The listing builds one solid part. Answer for the finished solid, in the listing's coordinates (mm). Face numbers are marked on the shaded views. A direction names the side the tool comes from. Coordinates: 2 decimals unless noted, no trailing zeros. Loops run counter-clockwise (first coordinate to the right, second up) from the corner with the lowest first, then second, coordinate; pieces in that order, holes last. Notation, with made-up numbers: (70, 34.5) -> (129, 34.5) arc R7 ccw to (129, 39.5) -> close; hole circle Ø6 at (-16, -29). An arc over 180 degrees is marked (long way). Answer in a Markdown table with one row per item.
```python
from build123d import *

# Parameters (mm, degrees)
BOSS_EXTRUDE1_DEPTH = 2.5
SKETCH2_R           = 1
CUT_EXTRUDE1_DEPTH  = 4.5
SKETCH3_R           = 1
CUT_EXTRUDE2_DEPTH  = 9.5
SKETCH5_R           = 1
BOSS_EXTRUDE2_DEPTH = 9.5
SKETCH7_W           = 2.5
SKETCH7_H           = 2.48697386
BOSS_EXTRUDE5_DEPTH = 17
SKETCH8_R           = 1
CUT_EXTRUDE3_DEPTH  = 9.5
SKETCH9_W           = 2.5
SKETCH9_H           = 2.510853282
CUT_EXTRUDE4_DEPTH  = 10.5
SKETCH10_R          = 1
CUT_EXTRUDE5_DEPTH  = 4.5
SKETCH11_R          = 1
BOSS_EXTRUDE6_DEPTH = 4.5
SKETCH12_R          = 1
CUT_EXTRUDE6_DEPTH  = 4
SKETCH13_W          = 2.5
SKETCH13_H          = 2.5
CUT_EXTRUDE7_DEPTH  = 6.5
SKETCH14_W          = 2.5
SKETCH14_H          = 2.5
BOSS_EXTRUDE7_DEPTH = 6.5
SKETCH15_R          = 1
CUT_EXTRUDE8_DEPTH  = 5


with BuildPart() as part:
    # Sketch1 → Boss-Extrude1 (new body)
    with BuildSketch(Plane.XY):
        Polygon((-70.406172668, -77.710060133), (-55.350496572, -77.710060133), (-55.155758053, -77.477979804), (-53.240646945, -79.084948828), (-54.184487309, -80.209773972), (-70.368347793, -80.209773972), align=None)
    extrude(amount=BOSS_EXTRUDE1_DEPTH)

    # Sketch2 → Cut-Extrude1 (cut)
    with BuildSketch(Plane(origin=(-60.939488189, -72.62485398, 0), x_dir=(0, 0, -1), z_dir=(0.6427876096865354, 0.7660444431189815, 0))):
        with Locations(Location((-1.25, -8.800123479, 0), (0, 0, 90))):
            Circle(SKETCH2_R)
    extrude(amount=-CUT_EXTRUDE1_DEPTH, mode=Mode.SUBTRACT)

    # Sketch3 → Cut-Extrude2 (cut)
    with BuildSketch(Plane(origin=(-71.565670343, -1.082908957, 0), x_dir=(0, 0, 1), z_dir=(-0.9998855357578962, -0.015129949839474955, 0))):
        with Locations(Location((1.25, -77.885923249, 0), (0, 0, 270))):
            Circle(SKETCH3_R)
    extrude(amount=-CUT_EXTRUDE2_DEPTH, mode=Mode.SUBTRACT)

    # Sketch5 → Boss-Extrude2 (add)
    with BuildSketch(Plane(origin=(-71.565670343, -1.082908957, 0), x_dir=(0, 0, 1), z_dir=(-0.9998855357578961, -0.015129949839476386, 0))):
        with Locations((1.25, -77.885923249)):
            Circle(SKETCH5_R)
    extrude(amount=-BOSS_EXTRUDE2_DEPTH)

    # Sketch7 → Boss-Extrude5 (add)
    with BuildSketch(Plane(origin=(-71.565670343, -1.082908957, 0), x_dir=(0, 0, 1), z_dir=(-0.9998855357578961, -0.015129949839476386, 0))):
        with Locations((1.25, -77.879410179)):
            Rectangle(SKETCH7_W, SKETCH7_H)
    extrude(amount=BOSS_EXTRUDE5_DEPTH)

    # Sketch8 → Cut-Extrude3 (cut)
    with BuildSketch(Plane(origin=(-88.56372445, -1.340118104, 0), x_dir=(0, 0, 1), z_dir=(-0.9998855357578962, -0.015129949839480206, 0))):
        with Locations(Location((1.25, -77.885923249, 0), (0, 0, 270))):
            Circle(SKETCH8_R)
    extrude(amount=-CUT_EXTRUDE3_DEPTH, mode=Mode.SUBTRACT)

    # Sketch9 → Cut-Extrude4 (cut)
    with BuildSketch(Plane(origin=(-88.56372445, -1.340118104, 0), x_dir=(0, 0, 1), z_dir=(-0.9998855357578962, -0.015129949839480206, 0))):
        with Locations((1.25, -77.89134989)):
            Rectangle(SKETCH9_W, SKETCH9_H)
    extrude(amount=-CUT_EXTRUDE4_DEPTH, mode=Mode.SUBTRACT)

    # Sketch10 → Cut-Extrude5 (cut)
    with BuildSketch(Plane(origin=(-78.064926325, -1.181253631, 0), x_dir=(0, 0, 1), z_dir=(-0.9998855357578961, -0.015129949839478678, 0))):
        with Locations(Location((1.25, -77.885923249, 0), (0, 0, 270))):
            Circle(SKETCH10_R)
    extrude(amount=-CUT_EXTRUDE5_DEPTH, mode=Mode.SUBTRACT)

    # Sketch11 → Boss-Extrude6 (add)
    with BuildSketch(Plane(origin=(-78.064926325, -1.181253631, 0), x_dir=(0, 0, 1), z_dir=(-0.9998855357578961, -0.015129949839478678, 0))):
        with Locations((1.25, -77.885923249)):
            Circle(SKETCH11_R)
    extrude(amount=-BOSS_EXTRUDE6_DEPTH)

    # Sketch12 → Cut-Extrude6 (cut)
    with BuildSketch(Plane(origin=(-78.064926325, -1.181253631, 0), x_dir=(0, 0, 1), z_dir=(-0.9998855357578961, -0.015129949839478678, 0))):
        with Locations(Location((1.25, -77.885923249, 0), (0, 0, 270))):
            Circle(SKETCH12_R)
    extrude(amount=-CUT_EXTRUDE6_DEPTH, mode=Mode.SUBTRACT)

    # Sketch13 → Cut-Extrude7 (cut)
    with BuildSketch(Plane(origin=(-78.064926325, -1.181253631, 0), x_dir=(0, 0, 1), z_dir=(-0.9998855357578961, -0.015129949839478678, 0))):
        with Locations((1.25, -77.885923249)):
            Rectangle(SKETCH13_W, SKETCH13_H)
    extrude(amount=-CUT_EXTRUDE7_DEPTH, mode=Mode.SUBTRACT)

    # Sketch14 → Boss-Extrude7 (add)
    with BuildSketch(Plane(origin=(-71.565670343, -1.082908957, 0), x_dir=(0, 0, 1), z_dir=(-0.9998855357578961, -0.015129949839476386, 0))):
        with Locations((1.25, -77.885923249)):
            Rectangle(SKETCH14_W, SKETCH14_H)
    extrude(amount=BOSS_EXTRUDE7_DEPTH)

    # Sketch15 → Cut-Extrude8 (cut)
    with BuildSketch(Plane(origin=(-78.064926325, -1.181253631, 0), x_dir=(0, 0, 1), z_dir=(-0.9998855357578961, -0.01512994983947622, 0))):
        with Locations(Location((1.25, -77.885923249, 0), (0, 0, 270))):
            Circle(SKETCH15_R)
    extrude(amount=-CUT_EXTRUDE8_DEPTH, mode=Mode.SUBTRACT)


solid = part.part
```
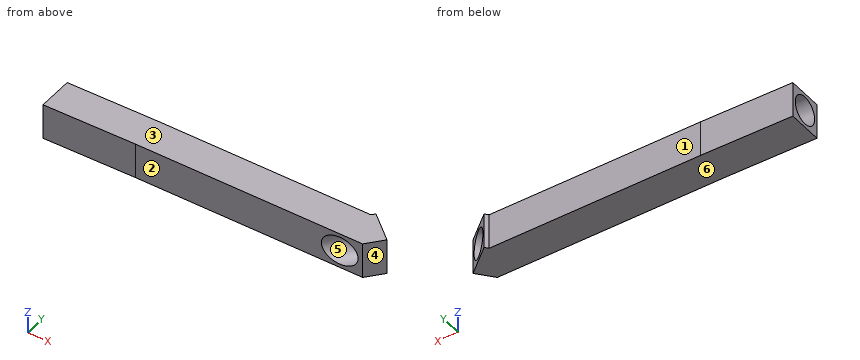
Item 1: A cutting plane is placed at C-C, the plane x = -71.25. Determine the outline of the cut face in (y, z), plus the area to 3 significant figures.
Findings below:
| item | result |
|---|---|
| outline | (-80.22, 0) -> (-77.72, 0) -> (-77.72, 2.5) -> (-80.22, 2.5) -> close |
| area | 6.25 mm2 |
Item 2: Find the intervals of material crossed by probe 1 along Y at (x, z) = (-61.5, 0.4); probe 2 along X at (y, z) = (-79.8, 0.4); probe 3 along X at (y, z) = (-79, 1.3), in increasing order.
Findings below:
| item | result |
|---|---|
| probe 1 | y = -80.21 to -77.71 |
| probe 2 | x = -76.88 to -56.16, -54.78 to -53.84 |
| probe 3 | x = -71.89 to -56.1, -53.5 to -53.34 |
Item 3: A cutting plane is placed at B-B, the plane x = -60.75. Determine the outline of the cut face in (y, z), plus the area to 3 significant figures.
Findings below:
| item | result |
|---|---|
| outline | (-80.21, 0) -> (-77.71, 0) -> (-77.71, 2.5) -> (-80.21, 2.5) -> close |
| area | 6.25 mm2 |
Item 4: A cutting plane is placed at A-A, the plane z = 0.55. Determine the outline of the cut face in (x, y), plus the area to 3 significant figures.
Findings below:
| item | result |
|---|---|
| outline | (-76.91, -77.81) -> (-76.9, -78.34) -> (-71.9, -78.27) -> (-71.88, -79.7) -> (-76.88, -79.77) -> (-76.87, -80.31) -> (-70.37, -80.21) -> (-56.75, -80.21) -> (-54.75, -77.82) -> (-55.16, -77.48) -> (-55.35, -77.71) -> (-70.41, -77.71) -> close; (-54.88, -80.21) -> (-54.18, -80.21) -> (-53.24, -79.08) -> (-53.65, -78.74) -> close |
| area | 46.8 mm2 |
Item 5: A tool of negligible diameter and unlimited length cuts with its end or side. For the marked faces 1, 2 and 3, from which of +Z, -Z, +X, -X, +Y, -Y can it reach the whole face along a straight path? Write none if from no direction.
Findings below:
| item | result |
|---|---|
| face 1 | +Z, -Z, -X, +Y |
| face 2 | +Z, -Z, +X, -Y |
| face 3 | +Z, +X, -X, +Y, -Y |
Item 6: Determine the mould class of the marked faces 4, 5 and 6 for opening direction X: +X half, -X half, draft (parallel to the pull), parting line (faces both ways), or undercut.
Findings below:
| item | result |
|---|---|
| face 4 | +X half |
| face 5 | undercut |
| face 6 | draft |
